```python
from build123d import *

# Parameters (mm, degrees)
F0_R     = 11.75
F1_DEPTH = 65
F3_DEPTH = 20
F4_R     = 5
F5_DEPTH = 13.501
F7_DEPTH = 45.001


with BuildPart() as f1:
    # F0 (on Front) → F1 (new body)
    with BuildSketch(Plane.XZ):
        Circle(F0_R)
    extrude(amount=F1_DEPTH)

    # F2 (on face) → F3 (cut)
    with BuildSketch(Plane.XZ.offset(65)):
        with BuildLine():
            ThreePointArc((11.61895, 1.75), (0, 11.75), (-11.61895, 1.75))
            Line((-11.61895, 1.75), (11.61895, 1.75))
        make_face()
    extrude(amount=-F3_DEPTH, mode=Mode.SUBTRACT)

    # F4 (on face) → F5 (cut, through all)
    with BuildSketch(Plane.XY.offset(1.75)):
        with Locations((0, -55)):
            Circle(F4_R)
    extrude(amount=-F5_DEPTH, mode=Mode.SUBTRACT)

    # F6 (on face) → F7 (cut, through all)
    with BuildSketch(Plane.XZ.offset(45)):
        with BuildLine():
            Line((-9.016035, 7.534827), (9.171855, 7.344357))
            ThreePointArc((9.171855, 7.344357), (0.123043, 11.749356), (-9.016035, 7.534827))
        make_face()
    extrude(amount=-F7_DEPTH, mode=Mode.SUBTRACT)


solid = f1.part
```
Geometry check sheet. Reference: the model listing, model coordinates, mm. A direction names the side the tool comes from. Coordinates: 2 decimals unless noted, no trailing zeros. Order: outer loops, then holes, each group sorted by start corner. A loop starts at its lowest first (then second) coordinate and runs counter-clockwise, first axis right, second up. Notation, with made-up numbers: (13.5, -18) - (33.5, -18) arc R15 cw to (33.5, 6) - close; hole circle Ø2 at (18, 11). An arc over 180 degrees is marked (long way). Answer in a Markdown table with one row per item. Add a question column.
1. Material ranges on L1, parallel to Y at x = 0, z = -3.5; L2, parallel to X at y = -55, z = -1; L3, parallel to X at y = -55, z = -5.5, recorded low to high. Write a range as [from, to].
2. Section check C-C (y = -55). Enter the section's corners in (x, z), plus the area to 3 significant figures.
3. Section check A-A (z = 0). Enter the section's corners in (x, y).
4. Access from +Z, -Z, +X, -X, +Y, -Y to the whole of each face (thin tool, end or side, straight path). Record for faces 4 (the face through (0, 0, -2)), 5 (the face through (-3, -60, 1.75)).
5. Section check D-D (y = -47). Enter the section's corners in (x, z), plus the area to 3 significant figures.
6. Draft check along X on faces 1 (the face through (-5, -55, -5)), 2 (the face through (-0.49, -32.04, -11.74)), 3 (the face through (0, -65, -3)). Enter one of: +X half, -X half, draft (parallel to the pull), parting line (faces both ways), or undercut.
7. Gauge pin test, flat ends, axial feed: pin 1 Ø10 at (x, y) = (-8.5, -38) entering from -Z; pin 2 Ø2 at (x, y) = (5, -55) entering from +Z; pin 3 Ø1 at (y, z) = (-10.5, -6.5) entering from +X. Record the tip position at first contact, or that the pin passes through.
8. Section check B-B (x = 0). Enter the section's corners in (y, z).
Data:
| question | item | result |
|---|---|---|
| 1 | L1 | y = [-65, -60], [-50, 0] |
| 1 | L2 | x = [-11.71, -5], [5, 11.71] |
| 1 | L3 | x = [-10.38, -5], [5, 10.38] |
| 2 | outline | (-11.62, 1.75) arc R11.75 ccw to (-5, -10.63) - (-5, 1.75) - close; (5, -10.63) arc R11.75 ccw to (11.62, 1.75) - (5, 1.75) - close |
| 2 | area | 126 mm² |
| 3 | outline | (-11.75, -65) - (11.75, -65) - (11.75, 0) - (-11.75, 0) - close; hole circle Ø10 at (0, -55) |
| 4 | face 4 | +Z, -Z, +X, -X, +Y |
| 4 | face 5 | +Z, +X, -X, -Y |
| 5 | outline | (-11.62, 1.75) arc R11.75 ccw (long way) to (11.62, 1.75) - close |
| 5 | area | 258 mm² |
| 6 | face 1 | undercut |
| 6 | face 2 | parting line |
| 6 | face 3 | draft |
| 7 | pin 1 | stops at z = -11.22 |
| 7 | pin 2 | stops at z = 1.75 |
| 7 | pin 3 | stops at x = 10.1 |
| 8 | outline | (-65, -11.75) - (-60, -11.75) - (-60, 1.75) - (-65, 1.75) - close; (-50, -11.75) - (0, -11.75) - (0, 7.44) - (-45, 7.44) - (-45, 1.75) - (-50, 1.75) - close |
